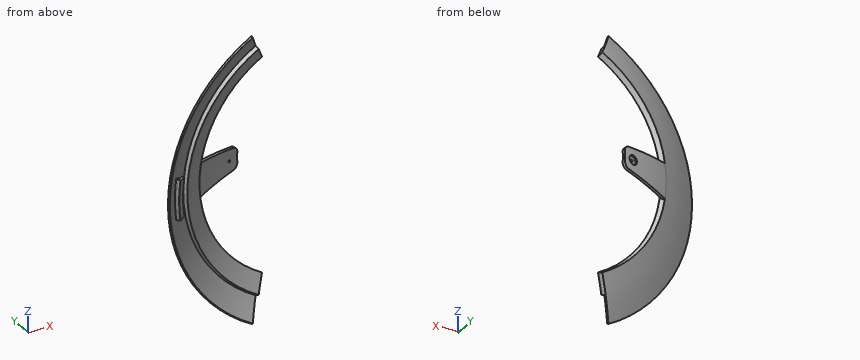
from build123d import *
from build123d.topology import SkipClean

# Parameters (mm, degrees)
REVOLVE2_ANGLE           = 60
REVOLVE2_OTHER_WAY_ANGLE = 60
REVOLVE3_ANGLE           = 8
REVOLVE3_OTHER_WAY_ANGLE = 8
FILLET1_R                = 5
CUT_REVOLVE1_START       = -250
CUT_REVOLVE1_OUTLINE_R   = 4
CUT_REVOLVE1_DEPTH       = 1.5
CUT_REVOLVE1_START_2     = -248.5
CUT_REVOLVE1_2_OUTLINE_R = 1
CUT_REVOLVE1_2_DEPTH     = 1.00202031
REVOLVE4_ANGLE           = 7.5
REVOLVE4_OTHER_WAY_ANGLE = 7.5


# Read off the part's stored shape, not the designer's step: Cut-Revolve1
with BuildPart() as part:
    # Sketch1 → Revolve2 (revolve)
    with BuildSketch(Plane.XY):
        with BuildLine():
            Line((-124.25, 215.20731284), (-122.5, 212.176223927))
            ThreePointArc((-122.5, 212.176223927), (-115.020532883, 216.32216025), (-107.400930963, 220.204541343))
            Line((-107.400930963, 220.204541343), (-109.592786697, 224.698511575))
            ThreePointArc((-109.592786697, 224.698511575), (-126.88459074, 215.40729011), (-143.394109088, 204.788011072))
            Line((-143.394109088, 204.788011072), (-142.533744433, 203.559283006))
            ThreePointArc((-142.533744433, 203.559283006), (-133.518952674, 209.582774284), (-124.25, 215.20731284))
        make_face()
    revolve(axis=Axis((0, 0, 0), (0, 1, 0)), revolution_arc=REVOLVE2_ANGLE)

    # Sketch1 → Revolve2 other way (revolve)
    with BuildSketch(Plane.XY):
        with BuildLine():
            Line((-124.25, 215.20731284), (-122.5, 212.176223927))
            ThreePointArc((-122.5, 212.176223927), (-115.020532883, 216.32216025), (-107.400930963, 220.204541343))
            Line((-107.400930963, 220.204541343), (-109.592786697, 224.698511575))
            ThreePointArc((-109.592786697, 224.698511575), (-126.88459074, 215.40729011), (-143.394109088, 204.788011072))
            Line((-143.394109088, 204.788011072), (-142.533744433, 203.559283006))
            ThreePointArc((-142.533744433, 203.559283006), (-133.518952674, 209.582774284), (-124.25, 215.20731284))
        make_face()
    revolve(axis=Axis((0, 0, 0), (0, -1, 0)), revolution_arc=REVOLVE2_OTHER_WAY_ANGLE)

    # Sketch2 → Revolve3 (revolve)
    with BuildSketch(Plane.XY):
        with BuildLine():
            ThreePointArc((-108.49685883, 222.451526459), (-86.676326862, 231.826366839), (-64.057713663, 239.066642007))
            Line((-64.057713663, 239.066642007), (-64.704761276, 241.481456572))
            ThreePointArc((-64.704761276, 241.481456572), (-87.551845315, 234.168047312), (-109.592786697, 224.698511575))
            Line((-109.592786697, 224.698511575), (-108.49685883, 222.451526459))
        make_face()
    revolve(axis=Axis((0, 0, 0), (0, 1, 0)), revolution_arc=REVOLVE3_ANGLE)

    # Sketch2 → Revolve3 other way (revolve)
    with BuildSketch(Plane.XY):
        with BuildLine():
            ThreePointArc((-108.49685883, 222.451526459), (-86.676326862, 231.826366839), (-64.057713663, 239.066642007))
            Line((-64.057713663, 239.066642007), (-64.704761276, 241.481456572))
            ThreePointArc((-64.704761276, 241.481456572), (-87.551845315, 234.168047312), (-109.592786697, 224.698511575))
            Line((-109.592786697, 224.698511575), (-108.49685883, 222.451526459))
        make_face()
    revolve(axis=Axis((0, 0, 0), (0, -1, 0)), revolution_arc=REVOLVE3_OTHER_WAY_ANGLE)

    # Fillet1
    fillet1_edges = [part.edges().sort_by_distance(p)[0] for p in [
        (-63.754683692, 240.274049289, -8.960136462),
        (-63.754683692, 240.274049289, 8.960136462),
    ]]
    fillet(fillet1_edges, radius=FILLET1_R)

    # Cut-Revolve1 outline → Cut-Revolve1 (cut)
    with SkipClean():  # the faces are left unmerged after this step: merging them gives an invalid solid
        with BuildSketch(Plane(origin=(0, 0, 0), x_dir=(0.9564822051761176, 0.29179066328693826, 0), z_dir=(0.2917906632869382, -0.9564822051761177, 0)).offset(CUT_REVOLVE1_START)):
            Circle(CUT_REVOLVE1_OUTLINE_R)
        extrude(amount=CUT_REVOLVE1_DEPTH, mode=Mode.SUBTRACT)

    # Cut-Revolve1 2 outline → Cut-Revolve1 2 (cut)
    with SkipClean():  # the faces are left unmerged after this step: merging them gives an invalid solid
        with BuildSketch(Plane(origin=(0, 0, 0), x_dir=(0.9564822051761176, 0.29179066328693826, 0), z_dir=(0.2917906632869382, -0.9564822051761177, 0)).offset(CUT_REVOLVE1_START_2)):
            Circle(CUT_REVOLVE1_2_OUTLINE_R)
        extrude(amount=CUT_REVOLVE1_2_DEPTH, mode=Mode.SUBTRACT)

    # Sketch4 → Revolve4 (revolve)
    with SkipClean():  # the faces are left unmerged after this step: merging them gives an invalid solid
        with BuildSketch(Plane.XY):
            with BuildLine():
                Line((-135.306423797, 208.433254735), (-134.48968482, 207.175106316))
                ThreePointArc((-134.48968482, 207.175106316), (-133.602565478, 207.748296017), (-132.713003262, 208.317687116))
                Line((-132.713003262, 208.317687116), (-133.518952674, 209.582774285))
                ThreePointArc((-133.518952674, 209.582774285), (-134.41391709, 209.009925345), (-135.306423797, 208.433254735))
            make_face()
            with BuildLine():
                Line((-134.48968482, 207.175106316), (-133.400699518, 205.497575091))
                ThreePointArc((-133.400699518, 205.497575091), (-132.520763328, 206.066123579), (-131.638404045, 206.630904224))
                Line((-131.638404045, 206.630904224), (-132.713003262, 208.317687116))
                ThreePointArc((-132.713003262, 208.317687116), (-133.602565478, 207.748296017), (-134.48968482, 207.175106316))
            make_face()
            with BuildLine():
                Line((-132.713003262, 208.317687116), (-131.638404045, 206.630904224))
                ThreePointArc((-131.638404045, 206.630904224), (-129.830219737, 207.771783558), (-128.012148355, 208.896840267))
                Line((-128.012148355, 208.896840267), (-129.057145485, 210.602120595))
                ThreePointArc((-129.057145485, 210.602120595), (-130.890058266, 209.467879751), (-132.713003262, 208.317687116))
            make_face()
        revolve(axis=Axis((0, 0, 0), (0, 1, 0)), revolution_arc=REVOLVE4_ANGLE)

    # Sketch4 → Revolve4 other way (revolve)
    with SkipClean():  # the faces are left unmerged after this step: merging them gives an invalid solid
        with BuildSketch(Plane.XY):
            with BuildLine():
                Line((-135.306423797, 208.433254735), (-134.48968482, 207.175106316))
                ThreePointArc((-134.48968482, 207.175106316), (-133.602565478, 207.748296017), (-132.713003262, 208.317687116))
                Line((-132.713003262, 208.317687116), (-133.518952674, 209.582774285))
                ThreePointArc((-133.518952674, 209.582774285), (-134.41391709, 209.009925345), (-135.306423797, 208.433254735))
            make_face()
            with BuildLine():
                Line((-134.48968482, 207.175106316), (-133.400699518, 205.497575091))
                ThreePointArc((-133.400699518, 205.497575091), (-132.520763328, 206.066123579), (-131.638404045, 206.630904224))
                Line((-131.638404045, 206.630904224), (-132.713003262, 208.317687116))
                ThreePointArc((-132.713003262, 208.317687116), (-133.602565478, 207.748296017), (-134.48968482, 207.175106316))
            make_face()
            with BuildLine():
                Line((-132.713003262, 208.317687116), (-131.638404045, 206.630904224))
                ThreePointArc((-131.638404045, 206.630904224), (-129.830219737, 207.771783558), (-128.012148355, 208.896840267))
                Line((-128.012148355, 208.896840267), (-129.057145485, 210.602120595))
                ThreePointArc((-129.057145485, 210.602120595), (-130.890058266, 209.467879751), (-132.713003262, 208.317687116))
            make_face()
        revolve(axis=Axis((0, 0, 0), (0, -1, 0)), revolution_arc=REVOLVE4_OTHER_WAY_ANGLE)


solid = part.part
Source: CAD feature listing. Evaluate the final solid. Frame: model axes, mm. Round coordinates to 2 decimals unless told otherwise and drop trailing zeros.
Q1. Section A-A, the plane x = -95.5. State how many separate pieces and enclosed holes the cut face has, plus the area to 3 significant figures.
Q2. Ray query, line 1 (Z direction, x = -85, y = 210); line 2 (X direction, y = 213.5, z = -75); line 3 (X direction, y = 208, z = -14). Return the intervals inside material, ascending.
Q3. First-contact query: P1, Ø1.5, axis at x = -91, y = 208.5, coming from the +Z side; P2, Ø10, axis at y = 207.5, z = -38, coming from the -X side; P3, Ø4, axis at y = 211.5, z = 84.5, coming from the -X side; P4, Ø5, axis at x = -115, y = 227, coming from the +Z side (3 decimals). Flat tips, straight axial feed; report the tip coordinate or a pass-through.
Solutions:
1. separate pieces: 3
1. enclosed holes: 0
1. area: 474 mm2
2. line 1: z = -105.71 to -102.11, 102.11 to 105.71
2. line 2: x = -106.27 to -102.69, -97.82 to -93.9
2. line 3: x = -137.99 to -135.25, -134.3 to -128.71
3. P1: stops at z = 105.3
3. P2: stops at x = -139.35
3. P3: stops at x = -107.4
3. P4: passes through
